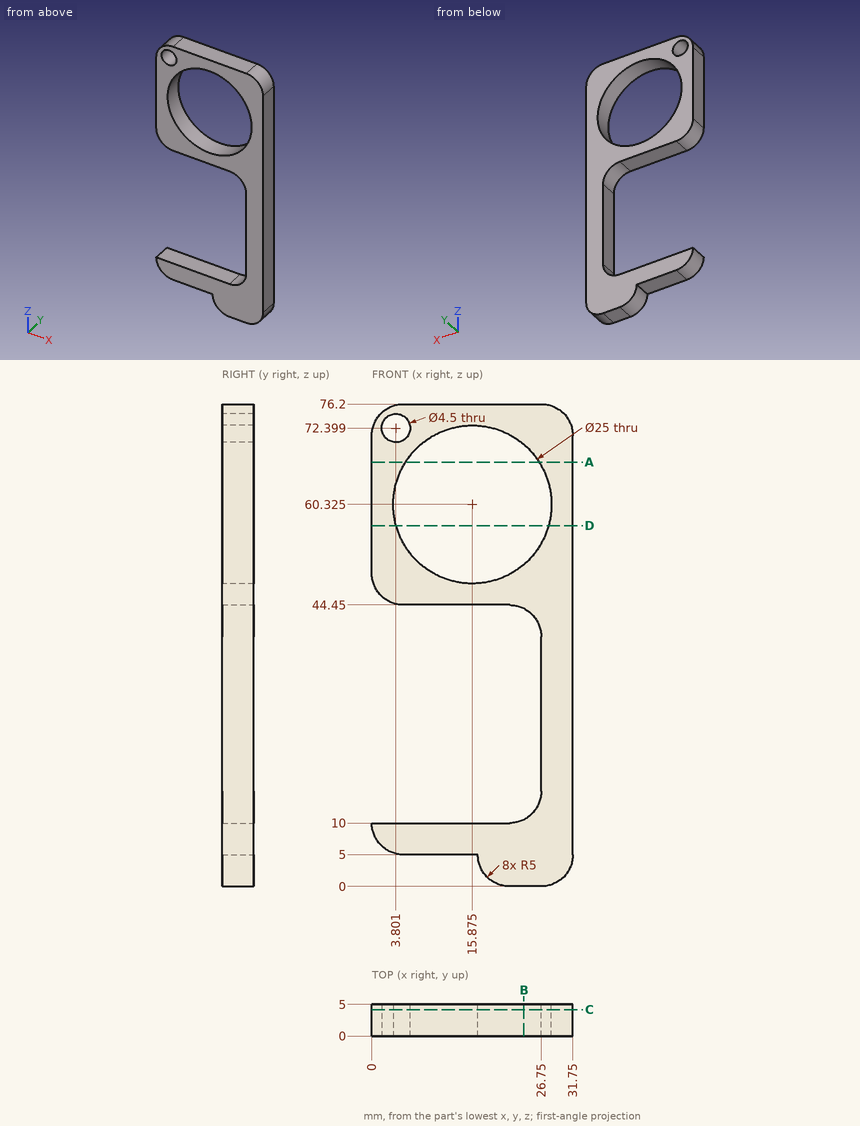
Check sheet for the drawn part. Datum: minimum x, y, z corner. Units: mm. Round coordinates to 2 decimals unless told otherwise and drop trailing zeros. Order: outer loops, then holes, each group sorted by start corner. A loop starts at its lowest first (then second) coordinate and runs counter-clockwise, first axis right, second up. Notation, with made-up numbers: (6, 19.25) -> (57, 19.25) arc R28 cw to (57, 49.25) -> close; hole circle Ø4 at (89, 5.5). An arc over 180 degrees is marked (long way). Put each result on its own line as item: value.
1) Depth check by flat-ended pin: pin 1 (2.5 mm diameter, centred on y = 2.5, z = 23.5, fed in from -X); pin 2 (1.5 mm diameter, centred on x = 13.5, y = 2.5, fed in from -Z). Enter the tip coordinate at first touch or a pass-through.
Final values:
pin 1: stops at x = 26.75
pin 2: stops at z = 5
2) Section check B-B (x = 24). Record the cut outline in (y, z), then the cut area to 3 significant figures.
Final values:
outline: (0, 0) -> (5, 0) -> (5, 10.53) -> (0, 10.53) -> close; (0, 43.92) -> (5, 43.92) -> (5, 50.83) -> (0, 50.83) -> close; (0, 69.82) -> (5, 69.82) -> (5, 76.2) -> (0, 76.2) -> close
area: 119 mm^2
3) Section check A-A (z = 67). Record the cut outline in (x, y), then the cut area to 3 significant figures.
Final values:
outline: (0, 0) -> (5.31, 0) -> (5.31, 5) -> (0, 5) -> close; (26.44, 0) -> (31.75, 0) -> (31.75, 5) -> (26.44, 5) -> close
area: 53.1 mm^2
4) Material ranges on line 1 (Z direction, x = 16.5, y = 3.25); line 2 (Z direction, x = 10, y = 3.45); line 3 (Z direction, x = 5.5, y = 0.9), recorded low to high.
Final values:
line 1: z = 5 to 10, 44.45 to 47.84, 72.81 to 76.2
line 2: z = 5 to 10, 44.45 to 49.29, 71.36 to 76.2
line 3: z = 5 to 10, 44.45 to 53.35, 67.3 to 70.92, 73.87 to 76.2
5) Section check D-D (z = 57). Record the cut outline in (x, y), then the cut area to 3 significant figures.
Final values:
outline: (0, 0) -> (3.83, 0) -> (3.83, 5) -> (0, 5) -> close; (27.92, 0) -> (31.75, 0) -> (31.75, 5) -> (27.92, 5) -> close
area: 38.3 mm^2
6) Section check C-C (y = 4.15). Record the cut outline in (x, z) (3 decimals), then the cut area to 3 significant figures.
Final values:
outline: (0, 10) arc R5 ccw to (5, 5) -> (16.75, 5) arc R5 ccw to (21.75, 0) -> (26.75, 0) arc R5 ccw to (31.75, 5) -> (31.75, 71.2) arc R5 ccw to (26.75, 76.2) -> (5, 76.2) arc R5 ccw to (0, 71.2) -> (0, 49.45) arc R5 ccw to (5, 44.45) -> (21.75, 44.45) arc R5 cw to (26.75, 39.45) -> (26.75, 15) arc R5 cw to (21.75, 10) -> close; hole circle Ø4.5 at (3.801, 72.399); hole circle Ø25 at (15.875, 60.325)
area: 886 mm^2
